```python
from build123d import *

# Parameters (mm, degrees)
CYLINDER_R     = 3.75
CYLINDER_DEPTH = 7
BOX_W          = 9.8
BOX_H          = 9.8
BOX_DEPTH      = 1


with BuildPart() as cilindro:
    # Cylinder → Cylinder (new body)
    with BuildSketch(Plane(origin=(5, 5, 0), x_dir=(1, 0, 0), z_dir=(0, 0, 1))):
        Circle(CYLINDER_R)
    extrude(amount=CYLINDER_DEPTH)


with BuildPart() as obj1:
    # Box → Box (new body)
    with BuildSketch(Plane(origin=(0.1, 0.1, 0), x_dir=(1, 0, 0), z_dir=(0, 0, 1))):
        with Locations((4.9, 4.9)):
            Rectangle(BOX_W, BOX_H)
    extrude(amount=BOX_DEPTH)

    # Fusion: union Cilindro
    add(cilindro.part)


solid = obj1.part
```
Here's how the part is built. I have some questions about the finished solid (model axes, mm). A direction names the side the tool comes from. Round coordinates to 2 decimals unless told otherwise and drop trailing zeros. Order: outer loops, then holes, each group sorted by start corner. A loop starts at its lowest first (then second) coordinate and runs counter-clockwise, first axis right, second up. Notation, with made-up numbers: (-10, -10.5) -> (10, -10.5) arc R24 ccw to (10, 1.5) -> close; hole circle Ø2 at (52.25, 39.5). An arc over 180 degrees is marked (long way). Use a Markdown table: item, result. Add a question column.
(1) I need wall thicknesses on line 1 along X through (y, z) = (5, 3.75); line 2 along Z through (x, y) = (1, 4.5); line 3 along X through (y, z) = (2.75, 4). Which ranges of each line are inside material? Lowest first, please.
(2) Suppose I cut it at D-D, the plane x = 9. Please give me the cut outline in (y, z).
(3) Suppose I cut it at C-C, the plane z = 2.5. Please give me the cut outline in (x, y), and give its area (3 significant figures).
(4) For pin 1 Ø2 at (y, z) = (5, 4) entering from -X; pin 2 Ø2 at (x, z) = (7.5, 3) entering from -Y, each with a flat end and sliding along its axis, tell me the tip position at first contact or that it passes through.
(5) Suppose I cut it at A-A, the plane x = 5. Please give me the cut outline in (y, z).
(6) For faces 1 (the face through (4.19, 1.34, 3.96)), 2 (the face through (0.1, 4.9, 0.5)), which set-ups out of +Z, -Z, +X, -X, +Y, -Y let a thin tool reach every point of the face, with its end or its side?
Verdict:
| question | item | result |
|---|---|---|
| 1 | line 1 | 1.25 to 8.75 |
| 1 | line 2 | 0 to 1 |
| 1 | line 3 | 2 to 8 |
| 2 | outline | (0.1, 0) -> (9.9, 0) -> (9.9, 1) -> (0.1, 1) -> close |
| 3 | outline | circle Ø7.5 at (5, 5) |
| 3 | area | 44.2 mm2 |
| 4 | pin 1 | x = 1.25 |
| 4 | pin 2 | y = 1.56 |
| 5 | outline | (0.1, 0) -> (9.9, 0) -> (9.9, 1) -> (8.75, 1) -> (8.75, 7) -> (1.25, 7) -> (1.25, 1) -> (0.1, 1) -> close |
| 6 | face 1 | +Z |
| 6 | face 2 | +Z, -Z, -X, +Y, -Y |
